```python
from build123d import *

# Parameters (mm, degrees)
SKETCH1_R           = 17.5
BOSS_EXTRUDE1_DEPTH = 41
FILLET2_R           = 1
SKETCH2_R           = 0.6
BOSS_EXTRUDE2_DEPTH = 5
FILLET3_R           = 0.5


with BuildPart() as part:
    # Sketch1 → Boss-Extrude1 (new body)
    with BuildSketch(Plane(origin=(0, 0, 0), x_dir=(1, 0, 0), z_dir=(0, 1, 0))):
        with Locations(Location((0, 0, 0), (0, 0, 270))):
            Circle(SKETCH1_R)
    extrude(amount=BOSS_EXTRUDE1_DEPTH)

    # Fillet2
    fillet2_edges = [part.edges().sort_by_distance(p)[0] for p in [
        (0, 41, -17.5),
    ]]
    fillet(fillet2_edges, radius=FILLET2_R)

    # Sketch2 → Boss-Extrude2 (add)
    with BuildSketch(Plane.XZ):
        with Locations(Location((0, 5, 0), (0, 0, 90))):
            Circle(SKETCH2_R)
        with Locations(Location((0, -5, 0), (0, 0, 90))):
            Circle(SKETCH2_R)
    extrude(amount=BOSS_EXTRUDE2_DEPTH)

    # Fillet3
    fillet3_edges = [part.edges().sort_by_distance(p)[0] for p in [
        (0, 0, -17.5),
    ]]
    fillet(fillet3_edges, radius=FILLET3_R)


solid = part.part
```
The model under review builds one solid part; all positions refer to its coordinate system, in mm. Round coordinates to 2 decimals unless told otherwise and drop trailing zeros. Write each loop counter-clockwise with the first axis right and the second up, starting at its lowest first coordinate (ties: lowest second). Pieces come first, ordered by that corner, then holes. Notation, with made-up numbers: (23, 0) - (49, 0) arc R9 ccw to (49, 17) - close; hole circle Ø3 at (72.25, -4). An arc over 180 degrees is marked (long way). Answer as CSV lines item,"result". Start each with the question number.
(1) Draft analysis for pull direction Z (two halves, no side actions). For faces 1 (the cylindrical face through (0, -2.5, 4.4)), 2 (the cylindrical face through (0, -2.5, -5.6)), 3 (the flat face through (0, -5, -5)), 4 (the cylindrical face through (-10.648, 19.974, -13.887)), state which applies: pulls with the +Z half, pulls with the -Z half, needs draft (parallel to the pull), parting line crosses it, or undercut.
(2) We need section B-B on x = 0. State the section outline as (y, z) points.
(3) We need section C-C on y = 17. State the section outline as (x, z) points, plus the area to 3 significant figures.
(4) We need section A-A on z = 0. State the section outline as (x, y) points.
(5) For pin 1 Ø3 at (y, z) = (17, -8) entering from +X; pin 2 Ø1.5 at (x, y) = (5.5, 0) entering from -Z; pin 3 Ø10 at (y, z) = (10, 10) entering from +X; pin 4 Ø17 at (x, z) = (-3.5, 3) entering from -Y, all flat-tipped, find the tip position at first contact; note any pin that passes through.
(6) To check wall thickness, follow line 1 (Y direction, x = -11, z = -1); line 2 (X direction, y = 19.5, z = 0.5); line 3 (X direction, y = 25.5, z = 12.5). State the ranges of each line that lie inside material, in increasing order.
Worked answers:
1,face 1,"undercut"
1,face 2,"undercut"
1,face 3,"needs draft"
1,face 4,"parting line crosses it"
2,outline,"(-5, -5.6) - (0, -5.6) - (0, -17) arc R0.5 ccw to (0.5, -17.5) - (40, -17.5) arc R1 ccw to (41, -16.5) - (41, 16.5) arc R1 ccw to (40, 17.5) - (0.5, 17.5) arc R0.5 ccw to (0, 17) - (0, 5.6) - (-5, 5.6) - (-5, 4.4) - (0, 4.4) - (0, -4.4) - (-5, -4.4) - close"
3,outline,"circle Ø35 at (0, 0)"
3,area,"962 mm²"
4,outline,"(-17.5, 0.5) arc R0.5 ccw to (-17, 0) - (17, 0) arc R0.5 ccw to (17.5, 0.5) - (17.5, 40) arc R1 ccw to (16.5, 41) - (-16.5, 41) arc R1 ccw to (-17.5, 40) - close"
5,pin 1,"x = 16.25"
5,pin 2,"z = -16.8"
5,pin 3,"x = 16.77"
5,pin 4,"y = -5"
6,line 1,"0 to 41"
6,line 2,"-17.49 to 17.49"
6,line 3,"-12.25 to 12.25"
